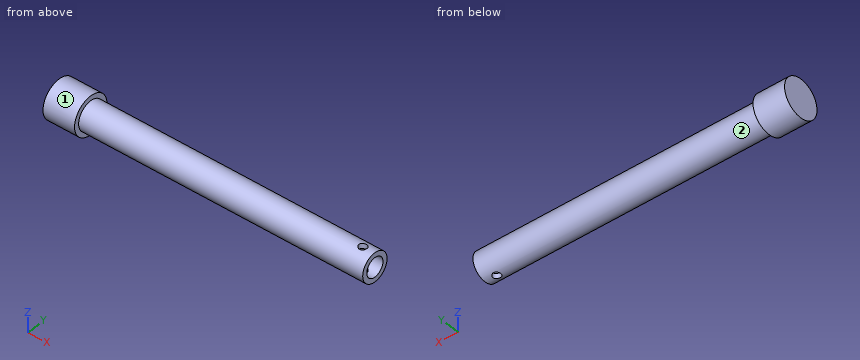
from build123d import *

# Parameters (mm, degrees)
SKETCH2_R               = 2.5
CUT_EXTRUDE1_DEPTH      = 13
CUT_EXTRUDE1_DEPTH_BACK = 13


with BuildPart() as part:
    # Sketch1 → Revolve1 (revolve)
    with BuildSketch(Plane.XY):
        Polygon((0, 0), (20, 0), (20, -6), (200, -6), (200, -9), (20, -9), (20, -12), (0, -12), align=None)
    revolve(axis=Axis((0, 0, 0), (1, 0, 0)))

    # Sketch2 → Cut-Extrude1 (cut, two sides)
    with BuildSketch(Plane.XY) as cut_extrude1_sk:
        with Locations((192.5, 0)):
            Circle(SKETCH2_R)
    extrude(amount=CUT_EXTRUDE1_DEPTH, mode=Mode.SUBTRACT)
    extrude(cut_extrude1_sk.sketch, amount=-CUT_EXTRUDE1_DEPTH_BACK, mode=Mode.SUBTRACT)


solid = part.part
Work out the finished part from the listing and answer in its coordinate system (mm). Face numbers are marked on the shaded views. A direction names the side the tool comes from. Round coordinates to 2 decimals unless told otherwise and drop trailing zeros. Loops run counter-clockwise (first coordinate to the right, second up) from the corner with the lowest first, then second, coordinate; pieces in that order, holes last. Notation, with made-up numbers: (52.25, 33.5) -> (71.25, 33.5) arc R20 cw to (71.25, 63.5) -> close; hole circle Ø5 at (12.5, -22). An arc over 180 degrees is marked (long way). Use one line per item in the form item = value.
(1) Straight lines are drawn through the part: line 1 (Z direction, x = 127, y = 0); line 2 (X direction, y = 0, z = -6.65). For each, find the intervals that lie inside material, in ascending order.
Answer list:
line_1 = -9 to -6, 6 to 9
line_2 = 0 to 190, 195 to 200
(2) Find section B-B on x = 192.5. Give the vertices of the cut face in (y, z), then the cut area to 3 significant figures.
Answer list:
outline = (-2.5, -8.65) -> (-2.5, -5.45) arc R6 cw to (-2.5, 5.45) -> (-2.5, 8.65) arc R9 ccw to start; (2.5, -8.65) arc R9 ccw to (2.5, 8.65) -> (2.5, 5.45) arc R6 cw to (2.5, -5.45) -> close
area = 111 mm2
(3) Find section D-D on x = 24. Give the vertices of the cut face in (y, z).
Answer list:
outline = circle Ø18 at (0, 0); hole circle Ø12 at (0, 0)
(4) Flat-ended cylindrical pins translate along their axes: P1, Ø3, axis at x = 58.5, z = 8, coming from the -Y side; P2, Ø10, axis at x = 80, y = -2.5, coming from the -Z side; P3, Ø4.5, axis at x = 192.5, y = 0, coming from the +Z side; P4, Ø4, axis at x = 135.5, z = 8.5, coming from the +Y side. Find the tip coordinate at first contact, or state that the pin passes through.
Answer list:
P1 = -6.22
P2 = -9
P3 = through
P4 = 6.22
(5) A tool of negligible diameter and unlimited length cuts with its end or side. For the marked faces 1 and 2, from which of +Z, -Z, +X, -X, +Y, -Y can it reach the whole face along a straight path? Write none if from no direction.
Answer list:
face_1 = +X, -X
face_2 = +X
(6) Find section C-C on z = 0. Give the vertices of the cut face in (x, y), then the cut area to 3 significant figures.
Answer list:
outline = (0, -12) -> (20, -12) -> (20, -9) -> (200, -9) -> (200, -6) -> (20, -6) -> (20, 6) -> (200, 6) -> (200, 9) -> (20, 9) -> (20, 12) -> (0, 12) -> close
area = 1,560 mm2
(7) Find section A-A on y = 0. Give the vertices of the cut face in (x, z).
Answer list:
outline = (0, -12) -> (20, -12) -> (20, -9) -> (190, -9) -> (190, -6) -> (20, -6) -> (20, 6) -> (190, 6) -> (190, 9) -> (20, 9) -> (20, 12) -> (0, 12) -> close; (195, -9) -> (200, -9) -> (200, -6) -> (195, -6) -> close; (195, 6) -> (200, 6) -> (200, 9) -> (195, 9) -> close
